Here's how the part is built. I have some questions about the finished solid (model axes, mm). A direction names the side the tool comes from. Coordinates: 2 decimals unless noted, no trailing zeros. Order: outer loops, then holes, each group sorted by start corner. A loop starts at its lowest first (then second) coordinate and runs counter-clockwise, first axis right, second up. Notation, with made-up numbers: (13.5, 37.5) - (36.5, 37.5) arc R25 cw to (36.5, 67.5) - close; hole circle Ø2 at (10, -21.5). An arc over 180 degrees is marked (long way). Answer as CSV lines item,"result". Start each with the question number.
Item 1: I need wall thicknesses on line 1 (X direction, y = 5.75, z = 0); line 2 (Z direction, x = -0.75, y = 10); line 3 (Z direction, x = -6, y = 16). Which ranges of each line are inside material? Lowest first, please.
Item 2: We'd pull the mould along Z, two halves only. Please class faces 1 (the face through (3.534, 42.797, 1.838)), 2 (the face through (9.1, 0, 3.3)), 3 (the face through (5.362, 5.413, 12.932)), 4 (the face through (-2.427, 23.648, -0.319)): pulls with the +Z half, pulls with the -Z half, needs draft (parallel to the pull), parting line crosses it, or undercut.
Item 3: On a 3-axis mill with a long thin cutter (end or side, diameter ignored), from which of +Z, -Z, +X, -X, +Y, -Y can I reach the whole of each face in a straight line? I mean faces 5 (the face through (7.59, 42.23, -1.69)), 6 (the face through (9.274, 5.916, -2.059)). Say none if no direction works.
Item 4: I'm going to push flat-ended pins straight in: pin 1 (3 mm diameter, centred on x = 8, z = -8.5, fed in from +Y); pin 2 (8 mm diameter, centred on x = 0.5, y = 54, fed in from -Z); pin 3 (8 mm diameter, centred on y = 15.5, z = 9.5, fed in from +X); pin 4 (5 mm diameter, centred on x = -5, z = -10.5, fed in from -Y). Where does each tip first touch, or does it pass through?
Item 5: Imagine slicing it at B-B on y = 34. List the corners of the cut face in (x, z) for me.
Item 6: Imagine slicing it at A-A on y = 18.5. List the corners of the cut face in (x, z) for me.
from build123d import *

# Parameters (mm, degrees)
FILLET1_R = 3


with BuildPart() as part:
    # Sketch1 → Revolve1 (revolve)
    with BuildSketch(Plane.XY, mode=Mode.PRIVATE) as revolve1_sk:
        with BuildLine():
            Line((9.5, 12), (9.5, 0))
            Line((9.5, 0), (14, 0))
            Line((14, 0), (14, 12))
            ThreePointArc((14, 12), (5.808899363, 24.991123715), (6.144902799, 40.3452934))
            Line((6.144902799, 40.3452934), (7.791407098, 41.20778213))
            Line((7.791407098, 41.20778213), (7.764668615, 42.858630405))
            Line((7.764668615, 42.858630405), (3.791041614, 42.794270306))
            ThreePointArc((3.791041614, 42.794270306), (3.509684474, 42.923205602), (3.394593546, 43.210503755))
            Line((3.394593546, 43.210503755), (3.39171112, 43.388466278))
            ThreePointArc((3.39171112, 43.388466278), (3.427062825, 43.564311584), (3.532381916, 43.709498374))
            ThreePointArc((3.532381916, 43.709498374), (6.047939548, 46.800239445), (6.141308054, 50.784206425))
            ThreePointArc((6.141308054, 50.784206425), (3.673190764, 56.254323111), (0, 61))
            Line((0, 61), (0, 27.143900008))
            Line((0, 27.143900008), (8.595760221, 14.867882182))
            ThreePointArc((8.595760221, 14.867882182), (9.268584754, 13.503528998), (9.5, 12))
        make_face()
    revolve(revolve1_sk.sketch.rotate(Axis((0, 61, 0), (0, -1, 0)), 90), axis=Axis((0, 61, 0), (0, -1, 0)))

    # Fillet1
    fillet1_edges = [part.edges().sort_by_distance(p)[0] for p in [
        (0, 12, -14),
    ]]
    fillet(fillet1_edges, radius=FILLET1_R)


solid = part.part
Responses:
1,line 1,"x = -14 to -9.5, 9.5 to 14"
1,line 2,"z = -13.98 to -9.47, 9.47 to 13.98"
1,line 3,"z = -8.32 to -4.99, 4.99 to 8.32"
2,face 1,"undercut"
2,face 2,"needs draft"
2,face 3,"parting line crosses it"
2,face 4,"undercut"
3,face 5,"+Y"
3,face 6,"-Y"
4,pin 1,"stops at y = 16.12"
4,pin 2,"stops at z = -6.33"
4,pin 3,"stops at x = 11.51"
4,pin 4,"stops at y = 0"
5,outline,"circle Ø9.82 at (0, 0)"
6,outline,"circle Ø17.15 at (0, 0); hole circle Ø12.11 at (0, 0)"
